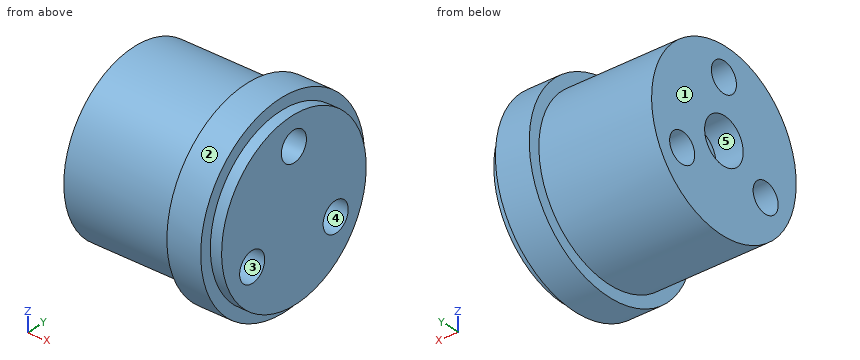
```python
from build123d import *

# Parameters (mm, degrees)
SKETCH102_R     = 1.3
POCKET010_DEPTH = 20
SKETCH103_R     = 2
POCKET011_DEPTH = 2.4


with BuildPart() as part:
    # Sketch101 → Revolution (revolve)
    with BuildSketch(Plane.XZ):
        Polygon((0, 0), (0, 7.5), (10, 7.5), (10, 8.5), (13, 8.5), (13, 7.5), (14, 7.5), (14, 0), align=None)
    revolve(axis=Axis((0, 0, 0), (1, 0, 0)))

    # Sketch102 (on DatumPlane) → Pocket010 (cut)
    with BuildSketch(Plane(origin=(0, 0, 0), x_dir=(0, 0, -1), z_dir=(-1, 0, 0))):
        with Locations((-5, 0)):
            Circle(SKETCH102_R)
        with Locations((2.5, -4.330127)):
            Circle(SKETCH102_R)
        with Locations((2.5, 4.330127)):
            Circle(SKETCH102_R)
    extrude(amount=-POCKET010_DEPTH, mode=Mode.SUBTRACT)

    # Sketch103 (on DatumPlane) → Pocket011 (cut)
    with BuildSketch(Plane(origin=(0, 0, 0), x_dir=(0, 0, -1), z_dir=(-1, 0, 0))):
        Circle(SKETCH103_R)
    extrude(amount=-POCKET011_DEPTH, mode=Mode.SUBTRACT)


solid = part.part
```
For this review, take the finished solid that the model builds, in its own axes (mm). Face numbers are marked on the shaded views. A direction names the side the tool comes from. Coordinates: 2 decimals unless noted, no trailing zeros. Write each loop counter-clockwise with the first axis right and the second up, starting at its lowest first coordinate (ties: lowest second). Pieces come first, ordered by that corner, then holes. Notation, with made-up numbers: (65, 78) - (119, 78) arc R18 ccw to (119, 82) - close; hole circle Ø10 at (37, -40). An arc over 180 degrees is marked (long way). Answer in a Markdown table with one row per item. Add a question column.
Q1. We need section C-C, the plane z = 0. State the section outline as (x, y) points.
Q2. We need section D-D, the plane y = -5.25. State the section outline as (x, z) points, and give its area (3 significant figures).
Q3. For P1, Ø1.6, axis at y = 4.33, z = -2.5, coming from the +X side; P2, Ø2, axis at x = 11.5, z = -6, coming from the +Y side; P3, Ø6, axis at x = 11.5, y = 4, coming from the -Z side; P4, Ø1.2, axis at y = 0.5, z = 0, coming from the -X side, all flat-tipped, find the tip position at first contact; note any pin that passes through.
Q4. Tool access review of the marked faces 4 and 5: name each direction out of +Z, -Z, +X, -X, +Y, -Y from which nothing blocks a thin tool from reaching the whole face with its end or side.
Q5. Draft analysis for pull direction Z (two halves, no side actions). For the marked faces 1, 2 and 3, state which applies: +Z half, -Z half, draft (parallel to the pull), parting line (faces both ways), or undercut.
Q6. For probe 1 along Y at (x, z) = (7.75, -2.5); probe 2 along Z at (x, y) = (4.5, 0); probe 3 along Z at (x, y) = (5.75, -4.5), list the stretches that pass through material, from the lowest coordinate up.
Q7. We need section B-B, the plane z = 5. State the section outline as (x, y) points.
Q8. We need section A-A, the plane y = 0. State the section outline as (x, z) points.
Answer list:
| question | item | result |
|---|---|---|
| 1 | outline | (0, -7.5) - (10, -7.5) - (10, -8.5) - (13, -8.5) - (13, -7.5) - (14, -7.5) - (14, 7.5) - (13, 7.5) - (13, 8.5) - (10, 8.5) - (10, 7.5) - (0, 7.5) - (0, 2) - (2.4, 2) - (2.4, -2) - (0, -2) - close |
| 2 | outline | (0, -5.36) - (10, -5.36) - (10, -6.68) - (13, -6.68) - (13, -5.36) - (14, -5.36) - (14, -3.42) - (0, -3.42) - close; (0, -1.58) - (14, -1.58) - (14, 5.36) - (13, 5.36) - (13, 6.68) - (10, 6.68) - (10, 5.36) - (0, 5.36) - close |
| 2 | area | 132 mm2 |
| 3 | P1 | passes through |
| 3 | P2 | stops at y = 6.87 |
| 3 | P3 | stops at z = -8.44 |
| 3 | P4 | stops at x = 2.4 |
| 4 | face 4 | +X, -X |
| 4 | face 5 | -X |
| 5 | face 1 | draft |
| 5 | face 2 | parting line |
| 5 | face 3 | undercut |
| 6 | probe 1 | y = -7.07 to -5.63, -3.03 to 3.03, 5.63 to 7.07 |
| 6 | probe 2 | z = -7.5 to 3.7, 6.3 to 7.5 |
| 6 | probe 3 | z = -6 to -3.79, -1.21 to 6 |
| 7 | outline | (0, -5.59) - (10, -5.59) - (10, -6.87) - (13, -6.87) - (13, -5.59) - (14, -5.59) - (14, -1.3) - (0, -1.3) - close; (0, 1.3) - (14, 1.3) - (14, 5.59) - (13, 5.59) - (13, 6.87) - (10, 6.87) - (10, 5.59) - (0, 5.59) - close |
| 8 | outline | (0, -7.5) - (10, -7.5) - (10, -8.5) - (13, -8.5) - (13, -7.5) - (14, -7.5) - (14, 3.7) - (0, 3.7) - (0, 2) - (2.4, 2) - (2.4, -2) - (0, -2) - close; (0, 6.3) - (14, 6.3) - (14, 7.5) - (13, 7.5) - (13, 8.5) - (10, 8.5) - (10, 7.5) - (0, 7.5) - close |
